Geometry: final body of the model. Coordinates: model frame, mm. A direction names the side the tool comes from. Give positions to 0.01 mm unless a question says otherwise; leave off trailing zeros. Write each loop counter-clockwise with the first axis right and the second up, starting at its lowest first coordinate (ties: lowest second). Pieces come first, ordered by that corner, then holes.
Q1. Line query: L1, parallel to X at y = -4, z = 11. Output: solid intervals per line, ascending.
Q2. Cut plane A-A on y = -24. Return the cut outline in (x, z).
Q3. Draft query along X for faces 1 (the face through (38.1, -19, 0)), 2 (the face through (-1, -19, 19.05)), 3 (the face through (16, -19, 7.996)). Return one class per face: pulls with the +X half, pulls with the -X half, needs draft (parallel to the pull), parting line crosses it, or undercut.
Q4. Cut plane B-B on z = 12. Return the cut outline in (x, y).
Q5. Reachability of faces 4 (the face through (10.044, -19, 11)), 5 (the face through (-1, -38.1, 0)) from +Z, -Z, +X, -X, +Y, -Y: full face, straight path, thin tool, end or side. Return the list, or none.
```python
from build123d import *

# Parameters (mm, degrees)
F0_W     = 76.2
F0_H     = 38.1
F2_DEPTH = 38.1
F1_W     = 12.7
F1_H     = 6.35
F3_DEPTH = 64.516


with BuildPart() as f2:
    # F0 (on Front) → F2 (new body)
    with BuildSketch(Plane.XZ):
        Rectangle(F0_W, F0_H)
    extrude(amount=F2_DEPTH)

    # F1 (on face) → F3 (cut)
    with BuildSketch(Plane.XZ):
        with Locations((16.394343, 11.170578)):
            Rectangle(F1_W, F1_H)
    extrude(amount=F3_DEPTH, mode=Mode.SUBTRACT)


solid = f2.part
```
Data:
1. L1: x = -38.1 to 10.04, 22.74 to 38.1
2. outline: (-38.1, -19.05) - (38.1, -19.05) - (38.1, 19.05) - (-38.1, 19.05) - close; hole (10.04, 8) - (22.74, 8) - (22.74, 14.35) - (10.04, 14.35) - close
3. face 1: pulls with the +X half
3. face 2: needs draft
3. face 3: undercut
4. outline: (-38.1, -38.1) - (10.04, -38.1) - (10.04, 0) - (-38.1, 0) - close; (22.74, -38.1) - (38.1, -38.1) - (38.1, 0) - (22.74, 0) - close
5. face 4: +Y, -Y
5. face 5: +Z, -Z, +X, -X, -Y
